```python
from build123d import *

# Parameters (mm, degrees)
BOSS_EXTRUDE1_DEPTH = 5.715
CUT_EXTRUDE1_REACH  = 53.513
SKETCH2_R           = 16.5
CUT_EXTRUDE2_REACH  = 53.513
SKETCH3_W           = 25.4
SKETCH3_H           = 5.715
CUT_EXTRUDE4_REACH  = 53.513


with BuildPart() as part:
    # Sketch1 → Boss-Extrude1 (new body)
    with BuildSketch(Plane.XY):
        with BuildLine():
            Line((25.4, -19.05), (-25.4, -19.05))
            Line((-25.4, -19.05), (-25.4, 19.05))
            ThreePointArc((-25.4, 19.05), (0, 44.45), (25.4, 19.05))
            Line((25.4, 19.05), (25.4, -19.05))
        make_face()
    extrude(amount=BOSS_EXTRUDE1_DEPTH)

    # Sketch2 → Cut-Extrude1 (cut, up to next)
    with BuildSketch(Plane.XY.offset(5.715), mode=Mode.PRIVATE) as cut_extrude1_sk1:
        with Locations((0, 22.21484)):
            Circle(SKETCH2_R)
    cut_extrude1_tool1 = extrude(cut_extrude1_sk1.sketch, amount=-CUT_EXTRUDE1_REACH, mode=Mode.PRIVATE) & part.part
    add(cut_extrude1_tool1.solids().sort_by_distance((0, 22.21484, 5.715))[0], mode=Mode.SUBTRACT)

    # Sketch3 → Cut-Extrude2 (cut, up to next)
    with BuildSketch(Plane.XY.offset(5.715), mode=Mode.PRIVATE) as cut_extrude2_sk1:
        with Locations((0, -16.1925)):
            Rectangle(SKETCH3_W, SKETCH3_H)
    cut_extrude2_tool1 = extrude(cut_extrude2_sk1.sketch, amount=-CUT_EXTRUDE2_REACH, mode=Mode.PRIVATE) & part.part
    add(cut_extrude2_tool1.solids().sort_by_distance((0, -16.1925, 5.715))[0], mode=Mode.SUBTRACT)

    # Sketch5 → Cut-Extrude4 (cut, up to next)
    with BuildSketch(Plane.XY.offset(5.715), mode=Mode.PRIVATE) as cut_extrude4_sk1:
        Polygon((3.175, -6.985), (1.143, -6.985), (1.143, -13.335), (-1.143, -13.335), (-1.143, -6.985), (-3.175, -6.985), (-3.175, -4.445), (-1.143, -4.445), (-1.143, 0.635), (1.143, 0.635), (1.143, -4.445), (3.175, -4.445), align=None)
    cut_extrude4_tool1 = extrude(cut_extrude4_sk1.sketch, amount=-CUT_EXTRUDE4_REACH, mode=Mode.PRIVATE) & part.part
    add(cut_extrude4_tool1.solids().sort_by_distance((0, -6.194885, 5.715))[0], mode=Mode.SUBTRACT)


solid = part.part
```
Check sheet for the modelled part. Datum: model origin and axes. Units: mm. A direction names the side the tool comes from. Round coordinates to 2 decimals unless told otherwise and drop trailing zeros. Order: outer loops, then holes, each group sorted by start corner. A loop starts at its lowest first (then second) coordinate and runs counter-clockwise, first axis right, second up. Notation, with made-up numbers: (47.5, -3) -> (94.5, -3) arc R20 cw to (94.5, 34) -> close; hole circle Ø7 at (54.5, -28). An arc over 180 degrees is marked (long way). One line per item, written item: value. Start each with the question number.
Q1. Cross-section at C-C (z = 4.6). Record the boundary of the cut face in (x, y) (3 decimals).
Q2. Set-up check for faces 1 (the face through (2, -6.985, 3)), 2 (the face through (1.143, -10, 3)), 3 (the face through (6, 6, 0)): record each of +Z, -Z, +X, -X, +Y, -Y from which the full face is reachable in a straight line by a thin tool's end or side.
Q3. Mould release check, pull along X, two halves, no side actions. Record for faces 4 (the face through (19, -19.05, 3)), 5 (the face through (-2, -6.985, 3)), 6 (the face through (-25.4, 0, 3)): pulls with the +X half, pulls with the -X half, needs draft (parallel to the pull), parting line crosses it, or undercut.
Q4. Cross-section at B-B (y = 30.5). Record the boundary of the cut face in (x, z) (3 decimals), and give its area (3 significant figures).
Q5. Cross-section at A-A (x = 0). Record the boundary of the cut face in (y, z) (3 decimals).
Q6. Thickness scan on line 1 (Y direction, x = 0, z = 2.8) (3 decimals); line 2 (X direction, y = -8.5, z = 1.4); line 3 (Y direction, x = 2, z = 1.55) (1 decimal). Record the ranges inside material, lowest first.
Q7. Cross-section at D-D (x = 20.5). Record the boundary of the cut face in (y, z) (3 decimals), and give its area (3 significant figures).
Q8. Gauge pin test, flat ends, axial feed: pin 1 Ø1.6 at (x, z) = (-2.5, 3) entering from -Y (3 decimals); pin 2 Ø1.1 at (x, z) = (0.5, 2) entering from -Y (3 decimals); pin 3 Ø3 at (y, z) = (36, 3.5) entering from -X. Record the tip position at first contact, or that the pin passes through.
Completed:
1. outline: (-25.4, -19.05) -> (-12.7, -19.05) -> (-12.7, -13.335) -> (-1.143, -13.335) -> (-1.143, -6.985) -> (-3.175, -6.985) -> (-3.175, -4.445) -> (-1.143, -4.445) -> (-1.143, 0.635) -> (1.143, 0.635) -> (1.143, -4.445) -> (3.175, -4.445) -> (3.175, -6.985) -> (1.143, -6.985) -> (1.143, -13.335) -> (12.7, -13.335) -> (12.7, -19.05) -> (25.4, -19.05) -> (25.4, 19.05) arc R25.4 ccw to (-25.4, 19.05) -> close; hole circle Ø33 at (0, 22.215)
2. face 1: +Z, -Z
2. face 2: +Z, -Z, -Y
2. face 3: -Z, +X, -X, +Y, -Y
3. face 4: needs draft
3. face 5: undercut
3. face 6: pulls with the -X half
4. outline: (-22.673, 0) -> (-14.269, 0) -> (-14.269, 5.715) -> (-22.673, 5.715) -> close; (14.269, 0) -> (22.673, 0) -> (22.673, 5.715) -> (14.269, 5.715) -> close
4. area: 96.1 mm²
5. outline: (0.635, 0) -> (5.715, 0) -> (5.715, 5.715) -> (0.635, 5.715) -> close; (38.715, 0) -> (44.45, 0) -> (44.45, 5.715) -> (38.715, 5.715) -> close
6. line 1: y = 0.635 to 5.715, 38.715 to 44.45
6. line 2: x = -25.4 to -1.14, 1.14 to 25.4
6. line 3: y = -13.3 to -7, -4.4 to 5.8, 38.6 to 44.4
7. outline: (-19.05, 0) -> (34.047, 0) -> (34.047, 5.715) -> (-19.05, 5.715) -> close
7. area: 303 mm²
8. pin 1: stops at y = -13.335
8. pin 2: stops at y = 0.635
8. pin 3: stops at x = -20.16
